```python
from build123d import *

# Parameters (mm, degrees)
F0_R         = 1.6
F1_DEPTH     = 15
F2_DEPTH     = 2
F3_T1_DEPTH  = 23.52
F3_T3_DEPTH  = 23.52
F3_T5_DEPTH  = 23.52
F3_T7_DEPTH  = 23.52
F3_T9_DEPTH  = 23.52
F3_T11_DEPTH = 23.52
F3_T13_DEPTH = 23.52


# Not quite as in the source:
# - a fillet or chamfer that OpenCascade refuses, or shapes differently, is made with other operations: its cross-section is extruded or revolved along the edge and cut away or added


with BuildPart() as f1:
    # F0 (on Top) → F1 (new body)
    with BuildSketch(Plane.XY):
        with BuildLine():
            ThreePointArc((-2.858932117, 1.6276078), (-2.4589449365, 1.3214191477), (-2.071427552, 0.9995938658))
            ThreePointArc((-2.071427552, 0.9995938658), (-2.242334198, 0.5117981481), (-2.2999992606, -0.0018442221))
            ThreePointArc((-2.2999992606, -0.0018442221), (-2.7887751164, -0.1236612902), (-3.2820013909, -0.2259798001))
            Line((-3.2820013909, -0.2259798001), (-3.0550300383, -1.2204062706))
            ThreePointArc((-3.0550300383, -1.2204062706), (-2.5662541825, -1.0985892024), (-2.073027908, -0.9962706925))
            ThreePointArc((-2.073027908, -0.9962706925), (-1.7982124097, -1.4340265443), (-1.4325842124, -1.7993616853))
            ThreePointArc((-1.4325842124, -1.7993616853), (-1.6420905549, -2.2574537369), (-1.8696162748, -2.7068681137))
            Line((-1.8696162748, -2.7068681137), (-0.9506280295, -3.1494295276))
            ThreePointArc((-0.9506280295, -3.1494295276), (-0.741121687, -2.691337476), (-0.5135959671, -2.2419230992))
            ThreePointArc((-0.5135959671, -2.2419230992), (0, -2.3), (0.5135959671, -2.2419230992))
            ThreePointArc((0.5135959671, -2.2419230992), (0.9979326, -2.0722283962), (1.4325842124, -1.7993616853))
            ThreePointArc((1.4325842124, -1.7993616853), (1.7982124097, -1.4340265443), (2.073027908, -0.9962706925))
            ThreePointArc((2.073027908, -0.9962706925), (2.242334198, -0.5117981481), (2.2999992606, -0.0018442221))
            ThreePointArc((2.2999992606, -0.0018442221), (2.242334198, 0.5117981481), (2.071427552, 0.9995938658))
            ThreePointArc((2.071427552, 0.9995938658), (2.4589449365, 1.3214191477), (2.858932117, 1.6276078))
            Line((2.858932117, 1.6276078), (2.2229725191, 2.4250759121))
            ThreePointArc((2.2229725191, 2.4250759121), (1.8354551346, 2.1032506302), (1.4354679542, 1.797061978))
            ThreePointArc((1.4354679542, 1.797061978), (0.9979326, 2.0722283962), (0.51, 2.2427438552))
            ThreePointArc((0.51, 2.2427438552), (0.5, 2.7463719276), (0.51, 3.25))
            Line((0.51, 3.25), (-0.51, 3.25))
            ThreePointArc((-0.51, 3.25), (-0.5, 2.7463719276), (-0.51, 2.2427438552))
            ThreePointArc((-0.51, 2.2427438552), (-0.9979326, 2.0722283962), (-1.4354679542, 1.797061978))
            ThreePointArc((-1.4354679542, 1.797061978), (-1.8354551346, 2.1032506302), (-2.2229725191, 2.4250759121))
            Line((-2.2229725191, 2.4250759121), (-2.858932117, 1.6276078))
        make_face()
        Circle(F0_R, mode=Mode.SUBTRACT)
        with BuildLine():
            ThreePointArc((2.2999992606, -0.0018442221), (2.242334198, -0.5117981481), (2.073027908, -0.9962706925))
            ThreePointArc((2.073027908, -0.9962706925), (2.5662541825, -1.0985892024), (3.0550300383, -1.2204062706))
            Line((3.0550300383, -1.2204062706), (3.2820013909, -0.2259798001))
            ThreePointArc((3.2820013909, -0.2259798001), (2.7887751164, -0.1236612902), (2.2999992606, -0.0018442221))
        make_face()
        with BuildLine():
            ThreePointArc((1.4325842124, -1.7993616853), (0.9979326, -2.0722283962), (0.5135959671, -2.2419230992))
            ThreePointArc((0.5135959671, -2.2419230992), (0.741121687, -2.691337476), (0.9506280295, -3.1494295276))
            Line((0.9506280295, -3.1494295276), (1.8696162748, -2.7068681137))
            ThreePointArc((1.8696162748, -2.7068681137), (1.6420905549, -2.2574537369), (1.4325842124, -1.7993616853))
        make_face()
    extrude(amount=F1_DEPTH)

    # F0 (on Top) → F2 (join)
    with BuildSketch(Plane.XY):
        Circle(F0_R)
    extrude(amount=F2_DEPTH)

    # F3: fillet of radius 4.5 on 7 edges, made by hand

    # F3_s2 → F3_t1 (cut)
    with BuildSketch(Plane(origin=(-10.5953938865, -5.102472772, 0), x_dir=(0, 0, 1), z_dir=(0.9009688679, 0.4338837391, 0))):
        with BuildLine():
            ThreePointArc((0, -1.25), (1.3180194847, 1.9319805153), (4.5, 3.25))
            Line((4.5, 3.25), (0, 3.25))
            Line((0, 3.25), (0, -1.25))
        make_face()
    extrude(amount=F3_T1_DEPTH, mode=Mode.SUBTRACT)

    # F3_s4 → F3_t3 (cut)
    with BuildSketch(Plane(origin=(-10.5953938865, 5.102472772, 0), x_dir=(0, 0, 1), z_dir=(0.9009688679, -0.4338837391, 0))):
        with BuildLine():
            ThreePointArc((0, -1.25), (1.3180194847, 1.9319805153), (4.5, 3.25))
            Line((4.5, 3.25), (0, 3.25))
            Line((0, 3.25), (0, -1.25))
        make_face()
    extrude(amount=F3_T3_DEPTH, mode=Mode.SUBTRACT)

    # F3_s6 → F3_t5 (cut)
    with BuildSketch(Plane(origin=(-2.6168461833, 11.4651522473, 0), x_dir=(0, 0, 1), z_dir=(0.222520934, -0.9749279122, 0))):
        with BuildLine():
            ThreePointArc((0, -1.25), (1.3180194847, 1.9319805153), (4.5, 3.25))
            Line((4.5, 3.25), (0, 3.25))
            Line((0, 3.25), (0, -1.25))
        make_face()
    extrude(amount=F3_T5_DEPTH, mode=Mode.SUBTRACT)

    # F3_s8 → F3_t7 (cut)
    with BuildSketch(Plane(origin=(7.3322400699, 9.1943382338, 0), x_dir=(0, 0, 1), z_dir=(-0.6234898019, -0.7818314825, 0))):
        with BuildLine():
            ThreePointArc((4.5, 3.25), (1.3180194847, 1.9319805153), (0, -1.25))
            Line((0, -1.25), (0, 3.25))
            Line((0, 3.25), (4.5, 3.25))
        make_face()
    extrude(amount=F3_T7_DEPTH, mode=Mode.SUBTRACT)

    # F3_s10 → F3_t9 (cut)
    with BuildSketch(Plane.YZ.offset(-11.76)):
        with BuildLine():
            ThreePointArc((-1.25, 0), (1.9319805153, 1.3180194847), (3.25, 4.5))
            Line((3.25, 4.5), (3.25, 0))
            Line((3.25, 0), (-1.25, 0))
        make_face()
    extrude(amount=F3_T9_DEPTH, mode=Mode.SUBTRACT)

    # F3_s12 → F3_t11 (cut)
    with BuildSketch(Plane(origin=(7.3322400699, -9.1943382338, 0), x_dir=(0, 0, 1), z_dir=(-0.6234898019, 0.7818314825, 0))):
        with BuildLine():
            ThreePointArc((0, -1.25), (1.3180194847, 1.9319805153), (4.5, 3.25))
            Line((4.5, 3.25), (0, 3.25))
            Line((0, 3.25), (0, -1.25))
        make_face()
    extrude(amount=F3_T11_DEPTH, mode=Mode.SUBTRACT)

    # F3_s14 → F3_t13 (cut)
    with BuildSketch(Plane(origin=(-2.6168461833, -11.4651522473, 0), x_dir=(0, 0, 1), z_dir=(0.222520934, 0.9749279122, 0))):
        with BuildLine():
            ThreePointArc((0, -1.25), (1.3180194847, 1.9319805153), (4.5, 3.25))
            Line((4.5, 3.25), (0, 3.25))
            Line((0, 3.25), (0, -1.25))
        make_face()
    extrude(amount=F3_T13_DEPTH, mode=Mode.SUBTRACT)


solid = f1.part
```
The listing builds one solid part. Answer for the finished solid, in the listing's coordinates (mm). A direction names the side the tool comes from. Give positions to 0.01 mm unless a question says otherwise; leave off trailing zeros. One line per item, written item: value.
1. For a pull along X with two mould halves and no side action, classify faces 3 (the face through (1.645, -2.264, 8.238)), 4 (the face through (-1.02, -2.086, 1.763)), 5 (the face through (2.559, -1.097, 8.238)) as pulls with the +X half, pulls with the -X half, needs draft (parallel to the pull), parting line crosses it, or undercut.
Found:
face 3: pulls with the +X half
face 4: pulls with the -X half
face 5: undercut
2. Find the intervals of material crossed by probe 1 along X at (y, z) = (2, 11.5); probe 2 along X at (y, z) = (2.5, 2.5); probe 3 along X at (y, z) = (0.5, 7.5) (3 decimals), in increasing order.
Found:
probe 1: -2.56 to -1.7, -1.14 to 1.14, 1.7 to 2.56
probe 2: -0.5 to 0.5
probe 3: -2.245 to -1.52, 1.52 to 2.245
3. Each of these flat-tipped pins is pushed along its axis until it touches: P1, Ø3, axis at y = 2.5, z = 12.5, coming from the -X side; P2, Ø1.5, axis at y = 0, z = 8.5, coming from the -X side; P3, Ø1, axis at y = -1.5, z = 11.5, coming from the -X side; P4, Ø1.6, axis at x = 0, y = -0.5, coming from the +Z side. Where does it stop, or does it pass through?
Found:
P1: x = -2.86
P2: x = -3.28
P3: x = -3.11
P4: z = 2
4. For faces 1 (the face through (-1.64, -2.25, 8.24)), 2 (the face through (-2.57, -1.1, 8.24)), determine the directions among +Z, -Z, +X, -X, +Y, -Y from which every point of the face is accessible in a straight line to the end or side of a thin tool.
Found:
face 1: +Z, -Z, -X
face 2: +Z, -Z, -Y
